The model under review builds one solid part; all positions refer to its coordinate system, in mm. Give positions to 0.01 mm unless a question says otherwise; leave off trailing zeros. Loops run counter-clockwise (first coordinate to the right, second up) from the corner with the lowest first, then second, coordinate; pieces in that order, holes last. Notation, with made-up numbers: M 36.25,71 L 70.25,71 A16 ccw 70.25,84 Z; hole C -35,-4.5 d9. An arc over 180 degrees is marked long. One line per item, written item: value. Start each with the question number.
Q1. We need section A-A on y = 0. Write out the cut boundary in (x, z), plus the area to 3 significant figures.
Q2. For pin 1 (5 mm diameter, centred on x = 11.79, y = -11.79, fed in from +Z) (3 decimals); pin 2 (4 mm diameter, centred on x = -11.79, y = 11.79, fed in from -Z); pin 3 (2 mm diameter, centred on x = -6.5, z = 0.5, fed in from -Y), all flat-tipped, find the tip position at first contact; note any pin that passes through.
Q3. To check wall thickness, follow line 1 along Y through (x, z) = (13, 1.2); line 2 along X through (y, z) = (1, 0.9); line 3 along X through (y, z) = (-2.5, 0.2). State the ranges of each line that lie inside material, in increasing order. Write a range as from..to.
Q4. We need section C-C on x = 12. Write out the cut boundary in (y, z) (3 decimals).
Q5. Mouldability with a two-part tool opening along X and no side actions: class faces 1 (the face through (7.745, -15.599, 2.576)), 2 (the face through (-3.192, 24.307, 2.504)) as released by +X, released by -X, zero draft, split by the parting line, or undercut.
Q6. We need section D-D on z = 1.2. Give the number of separate pieces and of enclosed holes in the cut face, plus the area to 3 significant figures.
```python
from build123d import *

# Parameters (mm, degrees)
F0_R            = 24.51608
F0_R_2          = 2.15265
F0_R_3          = 11.1125
F1_DEPTH        = 5.08
F3_DEPTH        = 5.08
F3_COPIES_COUNT = 4
F4_R            = 0.762
F6_R            = 3.96875
F7_DEPTH        = 1.905


# Not quite as in the source:
# - a pattern or mirror of a feature is missing from the dataset's text; its kind, count and spacing are read off the source's solid


with BuildPart() as f1:
    # F0 (on Top) → F1 (new body)
    with BuildSketch(Plane.XY):
        Circle(F0_R)
        with Locations((-11.7865906, -11.7865906)):
            Circle(F0_R_2, mode=Mode.SUBTRACT)
        with Locations((11.7865906, -11.7865906)):
            Circle(F0_R_2, mode=Mode.SUBTRACT)
        with Locations((-11.7865906, 11.7865906)):
            Circle(F0_R_2, mode=Mode.SUBTRACT)
        Circle(F0_R_3, mode=Mode.SUBTRACT)
        with Locations((11.7865906, 11.7865906)):
            Circle(F0_R_2, mode=Mode.SUBTRACT)
    extrude(amount=F1_DEPTH)

    # F2 (on face) → F3 (cut, through all)
    with BuildSketch(Plane.XY.offset(5.08)):
        with BuildLine():
            ThreePointArc((-12.5005198818, 17.2967828873), (-8.5209455851, 16.2818633057), (-6.3255779254, 12.810921909))
            ThreePointArc((-6.3255779254, 12.810921909), (0, 14.2875), (6.3255779254, 12.810921909))
            ThreePointArc((6.3255779254, 12.810921909), (8.5209455851, 16.2818633057), (12.5005198818, 17.2967828873))
            ThreePointArc((12.5005198818, 17.2967828873), (0, 21.34108), (-12.5005198818, 17.2967828873))
        make_face()
    f3 = extrude(amount=-F3_DEPTH, mode=Mode.SUBTRACT)

    # F3_copies: F3 ×4 about axis
    f3_copies_axis = Axis((0, 0, 0), (0, 0, 1))
    for i in range(1, F3_COPIES_COUNT):
        add(f3.rotate(f3_copies_axis, i * 360 / F3_COPIES_COUNT), mode=Mode.SUBTRACT)

    # F4
    f4_edges = [f1.edges().sort_by_distance(p)[0] for p in [
        (-12.50052, 17.296783, 2.54),
        (12.50052, 17.296783, 2.54),
        (-17.296783, 12.50052, 2.54),
        (-17.296783, -12.50052, 2.54),
        (-12.50052, -17.296783, 2.54),
        (12.50052, -17.296783, 2.54),
        (17.296783, -12.50052, 2.54),
        (17.296783, 12.50052, 2.54),
    ]]
    fillet(f4_edges, radius=F4_R)

    # F6 (on face) → F7 (cut, through all)
    with BuildSketch(Plane.XY.offset(5.08)):
        with Locations((11.7865906, -11.7865906)):
            Circle(F6_R)
        with Locations((-11.7865906, 11.7865906)):
            Circle(F6_R)
    extrude(amount=-F7_DEPTH, mode=Mode.SUBTRACT)


solid = f1.part
```
Solved:
1. outline: M -24.52,0 L -21.34,0 L -21.34,5.08 L -24.52,5.08 Z; M -14.29,0 L -11.11,0 L -11.11,5.08 L -14.29,5.08 Z; M 11.11,0 L 14.29,0 L 14.29,5.08 L 11.11,5.08 Z; M 21.34,0 L 24.52,0 L 24.52,5.08 L 21.34,5.08 Z
1. area: 64.5 mm2
2. pin 1: z = 3.175
2. pin 2: through
2. pin 3: y = -23.89
3. line 1: -20.79..-13.56, -10.01..-6.36, -5.93..5.93, 6.36..10.01, 13.56..20.79
3. line 2: -24.5..-21.32, -14.25..-11.07, 11.07..14.25, 21.32..24.5
3. line 3: -24.39..-21.19, -14.07..-10.83, 10.83..14.07, 21.19..24.39
4. outline: M -21.378,0 L -13.929,0 L -13.929,3.175 L -15.75,3.175 L -15.75,5.08 L -21.378,5.08 Z; M -9.645,0 L 9.645,0 L 9.645,5.08 L -7.824,5.08 L -7.824,3.175 L -9.645,3.175 Z; M 13.929,0 L 21.378,0 L 21.378,5.08 L 13.929,5.08 Z
5. face 1: undercut
5. face 2: split by the parting line
6. separate pieces: 1
6. enclosed holes: 9
6. area: 950 mm2
